from build123d import *

# Parameters (mm, degrees)
SKETCH1_R           = 100
SKETCH1_R_2         = 14
SKETCH1_R_3         = 6.7
SKETCH1_R_4         = 6.9
BOSS_EXTRUDE1_DEPTH = 6
SKETCH1_3_R         = 110
SKETCH1_3_R_2       = 100
BOSS_EXTRUDE2_DEPTH = 80
BOSS_EXTRUDE3_START = -5
SKETCH1_10_R        = 17
SKETCH1_10_R_2      = 10.75
SKETCH1_10_R_3      = 10
SKETCH1_10_R_4      = 3
BOSS_EXTRUDE3_DEPTH = 5


with BuildPart() as part:
    # Sketch1 → Boss-Extrude1 (new body)
    with BuildSketch(Plane.XY):
        Circle(SKETCH1_R)
        with Locations((0, 65)):
            Circle(SKETCH1_R_2, mode=Mode.SUBTRACT)
        with Locations((-41.121809018, 65)):
            Circle(SKETCH1_R_3, mode=Mode.SUBTRACT)
        with Locations((41.121809018, 65)):
            Circle(SKETCH1_R_4, mode=Mode.SUBTRACT)
    extrude(amount=BOSS_EXTRUDE1_DEPTH)

    # Sketch1_3 → Boss-Extrude2 (add)
    with BuildSketch(Plane.XY):
        Circle(SKETCH1_3_R)
        Circle(SKETCH1_3_R_2, mode=Mode.SUBTRACT)
    extrude(amount=BOSS_EXTRUDE2_DEPTH)

    # Sketch1_10 → Boss-Extrude3 (add)
    # profile 1 of 3: a face of its own
    with BuildSketch(Plane.XY.offset(BOSS_EXTRUDE3_START)):
        with Locations((0, 65)):
            Circle(SKETCH1_10_R)
        with Locations((0, 65)):
            Circle(SKETCH1_10_R_2, mode=Mode.SUBTRACT)
    # profile 2 of 3: a face of its own
    with BuildSketch(Plane.XY.offset(BOSS_EXTRUDE3_START)):
        with Locations((41.121809018, 65)):
            Circle(SKETCH1_10_R_3)
        with BuildLine():
            ThreePointArc((48.021809018, 65), (41.121809018, 58.1), (34.221809018, 65))
            ThreePointArc((34.221809018, 65), (41.121809018, 71.9), (48.021809018, 65))
        make_face(mode=Mode.SUBTRACT)
    # profile 3 of 3: a face of its own
    with BuildSketch(Plane.XY.offset(BOSS_EXTRUDE3_START)):
        with Locations((-41.121809018, 65)):
            Circle(SKETCH1_10_R_3)
        with Locations((-41.121809018, 65)):
            Circle(SKETCH1_10_R_4, mode=Mode.SUBTRACT)
    extrude(amount=BOSS_EXTRUDE3_DEPTH)


solid = part.part
Verification items for the finished model (mm, model axes). A direction names the side the tool comes from. Give positions to 0.01 mm unless a question says otherwise; leave off trailing zeros. Write each loop counter-clockwise with the first axis right and the second up, starting at its lowest first coordinate (ties: lowest second). Pieces come first, ordered by that corner, then holes. Notation, with made-up numbers: (20.5, 78) - (52.5, 78) arc R15 cw to (52.5, 107) - close; hole circle Ø11 at (59.25, 45). An arc over 180 degrees is marked (long way). Answer as CSV lines item,"result". Start each with the question number.
1. Draft check along Y on faces 1 (the face through (-23.846, -107.384, 39.44)), 2 (the face through (-43.5, 62.9, -5)), 3 (the face through (-43.5, 63.17, -2.54)). Enter one of: pulls with the +Y half, pulls with the -Y half, needs draft (parallel to the pull), parting line crosses it, or undercut.
2. Sectioned sample at D-D (x = 96.5). Record the boundary of the cut face in (y, z), then the cut area to 3 significant figures.
3. Set-up check for faces 4 (the face through (4.1, 54.7, 0)), 5 (the face through (-3.685, 48.404, -2.535)), 6 (the face through (-2.3, 54.5, -2.5)): record each of +Z, -Z, +X, -X, +Y, -Y from which the full face is reachable in a straight line by a thin tool's end or side.
4. Sectioned sample at B-B (y = 0). Record the boundary of the cut face in (x, z), then the cut area to 3 significant figures.
5. Sectioned sample at A-A (x = 0). Record the boundary of the cut face in (y, z).
6. Depth check by flat-ended pin: pin 1 (1 mm diameter, centred on x = 77.5, z = 32, fed in from -Y); pin 2 (2 mm diameter, centred on y = 34.5, z = 32.5, fed in from -X); pin 3 (22.5 mm diameter, centred on x = 2, y = 60.5, fed in from +Z); pin 4 (11 mm diameter, centred on x = 41.12, y = 65, fed in from +Z). Enter the tip coordinate at first touch or a pass-through.
7. Thickness scan on line 1 (Y direction, x = 0, z = 1.35); line 2 (Y direction, x = 3, z = 68.5); line 3 (Z direction, x = 9.5, y = -40.5). Record the ranges inside material, lowest first.
8. Sectioned sample at C-C (z = 22.5). Record the boundary of the cut face in (x, y), then the cut area to 3 significant figures.
Derived:
1,face 1,"parting line crosses it"
1,face 2,"needs draft"
1,face 3,"undercut"
2,outline,"(-52.8, 0) - (52.8, 0) - (52.8, 80) - (26.22, 80) - (26.22, 6) - (-26.22, 6) - (-26.22, 80) - (-52.8, 80) - close"
2,area,"4,570 mm²"
3,face 4,"+Z"
3,face 5,"-Z"
3,face 6,"+Z, -Z"
4,outline,"(-110, 0) - (110, 0) - (110, 80) - (100, 80) - (100, 6) - (-100, 6) - (-100, 80) - (-110, 80) - close"
4,area,"2,800 mm²"
5,outline,"(-110, 0) - (48, 0) - (48, -5) - (54.25, -5) - (54.25, 0) - (51, 0) - (51, 6) - (-100, 6) - (-100, 80) - (-110, 80) - close; (75.75, -5) - (82, -5) - (82, 0) - (110, 0) - (110, 80) - (100, 80) - (100, 6) - (79, 6) - (79, 0) - (75.75, 0) - close"
6,pin 1,"y = -78.56"
6,pin 2,"x = -104.77"
6,pin 3,"z = 6"
6,pin 4,"through"
7,line 1,"-110 to 51, 79 to 110"
7,line 2,"-109.96 to -99.95, 99.95 to 109.96"
7,line 3,"0 to 6"
8,outline,"circle Ø220 at (0, 0); hole circle Ø200 at (0, 0)"
8,area,"6,600 mm²"
